from build123d import *

# Parameters (mm, degrees)
SKETCH2_W           = 10
SKETCH2_H           = 36
BOSS_EXTRUDE1_DEPTH = 2
SKETCH3_R           = 1
CUT_EXTRUDE1_DEPTH  = 2
SKETCH4_W           = 2
SKETCH4_H           = 36
BOSS_EXTRUDE2_DEPTH = 13
CUT_EXTRUDE2_DEPTH  = 10


with BuildPart() as part:
    # Sketch2 → Boss-Extrude1 (new body)
    with BuildSketch(Plane.XY):
        Rectangle(SKETCH2_W, SKETCH2_H)
    extrude(amount=BOSS_EXTRUDE1_DEPTH)

    # Sketch3 → Cut-Extrude1 (cut)
    with BuildSketch(Plane.XY.offset(2)):
        with Locations((0, 16)):
            Circle(SKETCH3_R)
        with Locations((0, -16)):
            Circle(SKETCH3_R)
    extrude(amount=-CUT_EXTRUDE1_DEPTH, mode=Mode.SUBTRACT)

    # Sketch4 → Boss-Extrude2 (add)
    with BuildSketch(Plane.XY.offset(2)):
        with Locations((-4, 0)):
            Rectangle(SKETCH4_W, SKETCH4_H)
    extrude(amount=BOSS_EXTRUDE2_DEPTH)

    # Sketch5 → Cut-Extrude2 (cut)
    with BuildSketch(Plane(origin=(-3, 0, 0), x_dir=(0, 0, -1), z_dir=(1, 0, 0))):
        with BuildLine():
            Line((-8, 13), (-8, -13))
            ThreePointArc((-8, -13), (-10, -15), (-12, -13))
            Line((-12, -13), (-12, 13))
            ThreePointArc((-12, 13), (-10, 15), (-8, 13))
        make_face()
    extrude(amount=-CUT_EXTRUDE2_DEPTH, mode=Mode.SUBTRACT)


solid = part.part
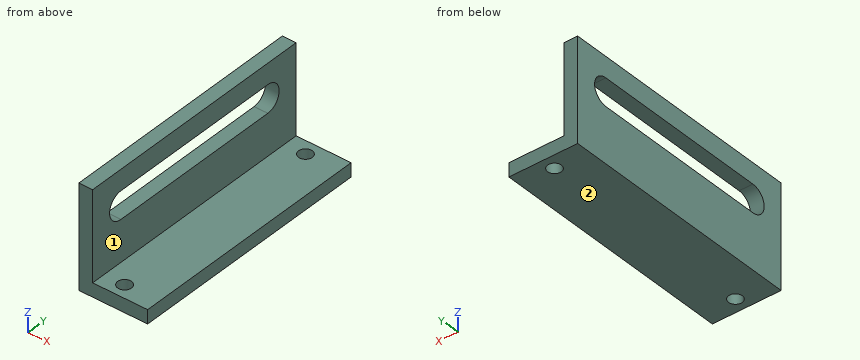
The listing builds one solid part. Answer for the finished solid, in the listing's coordinates (mm). Face numbers are marked on the shaded views. A direction names the side the tool comes from. Give positions to 0.01 mm unless a question says otherwise; leave off trailing zeros. Write each loop counter-clockwise with the first axis right and the second up, starting at its lowest first coordinate (ties: lowest second). Pieces come first, ordered by that corner, then holes.
1) A tool of negligible diameter and unlimited length cuts with its end or side. For the marked faces 1 and 2, from which of +Z, -Z, +X, -X, +Y, -Y can it reach the whole face along a straight path? Write none if from no direction.
2) Section A-A (y = 12) is taken. Write down the section's boundary in (x, z), and give its area (3 significant figures).
3) Find the intervals of material crossed by L1, parallel to Y at x = 0, z = 0.55; L2, parallel to Y at x = -0.5, z = 1; L3, parallel to X at y = 14, z = 5, in increasing order.
4) Section C-C (x = -0.25) is taken. Write down the section's boundary in (y, z).
5) Given P1, Ø0.6, axis at x = -4.5, y = 5.5, coming from the -Z side; P2, Ø1.5, axis at y = -13, z = 6.5, coming from the +X side; P3, Ø2.5, axis at x = 0, y = 16, coming from the +Z side, each flat-ended and moving along its own axis, determine where each tip first touches the part or whether it passes through.
6) Section D-D (y = -16) is taken. Write down the section's boundary in (x, z), and give its area (3 significant figures).
7) Section B-B (x = -4) is taken. Write down the section's boundary in (y, z), and give its area (3 significant figures).
Response:
1. face 1: +Z, +X, +Y, -Y
1. face 2: -Z, +X, -X, +Y, -Y
2. outline: (-5, 0) - (5, 0) - (5, 2) - (-3, 2) - (-3, 8) - (-5, 8) - close; (-5, 12) - (-3, 12) - (-3, 15) - (-5, 15) - close
2. area: 38.0 mm2
3. L1: y = -18 to -17, -15 to 15, 17 to 18
3. L2: y = -18 to -16.87, -15.13 to 15.13, 16.87 to 18
3. L3: x = -5 to -3
4. outline: (-18, 0) - (-16.97, 0) - (-16.97, 2) - (-18, 2) - close; (-15.03, 0) - (15.03, 0) - (15.03, 2) - (-15.03, 2) - close; (16.97, 0) - (18, 0) - (18, 2) - (16.97, 2) - close
5. P1: stops at z = 0
5. P2: stops at x = -3
5. P3: stops at z = 2
6. outline: (-5, 0) - (-1, 0) - (-1, 2) - (-3, 2) - (-3, 15) - (-5, 15) - close; (1, 0) - (5, 0) - (5, 2) - (1, 2) - close
6. area: 42.0 mm2
7. outline: (-18, 0) - (18, 0) - (18, 15) - (-18, 15) - close; hole (-13, 8) - (13, 8) arc R2 ccw to (13, 12) - (-13, 12) arc R2 ccw to start
7. area: 423 mm2
